Input: part model. Units: mm. Frame: model coordinates. Give positions to 0.01 mm unless a question says otherwise; leave off trailing zeros. Loops run counter-clockwise (first coordinate to the right, second up) from the corner with the lowest first, then second, coordinate; pieces in that order, holes last. Notation, with made-up numbers: (6, 66.25) - (35, 66.25) arc R20 ccw to (35, 75.25) - close; hole circle Ø5 at (50, 9). An arc over 180 degrees is marked (long way). Answer as a JSON object with one key per item and string values.
from build123d import *

# Parameters (mm, degrees)
BOSS_EXTRUDE2_DEPTH                          = 2
F_3_2_3_2_DIAMETER_HOLE1_D                   = 3.2
F_3_2_3_2_DIAMETER_HOLE2_D                   = 3.2
F_3_2_3_2_DIAMETER_HOLE3_D                   = 3.2
F_3_2_3_2_DIAMETER_HOLE5_D                   = 3.2
F_3_2_3_2_DIAMETER_HOLE5_DEPTH               = 10
F_3_2_3_2_DIAMETER_HOLE5_TIP                 = 0.96137699
CSK_FOR_M3_FLAT_COUNTERSUNK_HEAD_SCR_2_COUNT = 2
CSK_FOR_M3_FLAT_COUNTERSUNK_HEAD_SCR_2_PITCH = 78
CSK_FOR_M3_FLAT_COUNTERSUNK_HEAD_SCR_3_COUNT = 2
CSK_FOR_M3_FLAT_COUNTERSUNK_HEAD_SCR_3_PITCH = 110.308657865
FILLET1_R                                    = 3
M2_5X0_45_TAPPED_HOLE1_D                     = 2.05


with BuildPart() as part:
    # Sketch2 → Boss-Extrude2 (new body)
    with BuildSketch(Plane.ZY.offset(51.493641502)):
        Polygon((0.93465612, 3.45185693), (7.43465612, 3.45185693), (7.43465612, 86.45185693), (0.93465612, 86.45185693), (0.93465612, 92.95185693), (-82.06534388, 92.95185693), (-82.06534388, 86.45185693), (-88.56534388, 86.45185693), (-88.56534388, 3.45185693), (-82.06534388, 3.45185693), (-82.06534388, -3.04814307), (0.93465612, -3.04814307), align=None)
        Polygon((-71.56534388, 86.45185693), (-82.06534388, 75.95185693), (-82.06534388, 13.95185693), (-71.56534388, 3.45185693), (-9.56534388, 3.45185693), (0.93465612, 13.95185693), (0.93465612, 75.95185693), (-9.56534388, 86.45185693), align=None, mode=Mode.SUBTRACT)
    extrude(amount=BOSS_EXTRUDE2_DEPTH)

    # Sketch10 → CSK for M3 Flat Countersunk Head Screw3 (revolve, cut)
    with BuildSketch(Plane(origin=(-53.493641502, 5.95185693, -1.56534388), x_dir=(0, 0, 1), z_dir=(0, 1, 0))):
        Polygon((0, 0), (0, 2), (1.6, 2), (1.6, 1.65), (3.25, 0), align=None)
    revolve(axis=Axis((-59.843641502, 5.95185693, -1.56534388), (1, 0, 0)), mode=Mode.SUBTRACT)

    # Ø3.2 (3.2) Diameter Hole1 (through all)
    with Locations(Plane.ZY.offset(53.493641502)):
        with Locations((4.43465612, 6.95185693)):
            Hole(F_3_2_3_2_DIAMETER_HOLE1_D / 2)

    # Ø3.2 (3.2) Diameter Hole2 (through all)
    with Locations(Plane.ZY.offset(53.493641502)):
        with Locations((-2.56534388, -0.04814307)):
            Hole(F_3_2_3_2_DIAMETER_HOLE2_D / 2)

    # Ø3.2 (3.2) Diameter Hole3 (through all)
    with Locations(Plane.ZY.offset(53.493641502)):
        with Locations((-78.56534388, -0.04814307)):
            Hole(F_3_2_3_2_DIAMETER_HOLE3_D / 2)

    # Ø3.2 (3.2) Diameter Hole5
    with Locations(Plane(origin=(-53.493641502, 6.95185693, -85.56534388), x_dir=(0, 0, -1), z_dir=(-1, 0, 0))):
        with Locations((0, 0), (0, -76), (-7, -83), (-83, -83), (-90, -76)):
            Hole(F_3_2_3_2_DIAMETER_HOLE5_D / 2, depth=F_3_2_3_2_DIAMETER_HOLE5_DEPTH)
            with Locations((0, 0, -(F_3_2_3_2_DIAMETER_HOLE5_DEPTH + F_3_2_3_2_DIAMETER_HOLE5_TIP / 2))):  # 118° drill point
                Cone(0, F_3_2_3_2_DIAMETER_HOLE5_D / 2, F_3_2_3_2_DIAMETER_HOLE5_TIP, mode=Mode.SUBTRACT)

    # Sketch24 → CSK for M3 Flat Countersunk Head Screw5 (revolve, cut)
    with BuildSketch(Plane(origin=(-53.493641502, 5.95185693, -79.56534388), x_dir=(0, 0, 1), z_dir=(0, 1, 0))):
        Polygon((0, 0), (0, 2), (1.6, 2), (1.6, 1.65), (3.25, 0), align=None)
    csk_for_m3_flat_countersunk_head_screw5 = revolve(axis=Axis((-59.843641502, 5.95185693, -79.56534388), (1, 0, 0)), mode=Mode.SUBTRACT)

    # CSK for M3 Flat Countersunk Head Scr 2: CSK for M3 Flat Countersunk Head Screw5 ×2
    with Locations(*[(0, i * CSK_FOR_M3_FLAT_COUNTERSUNK_HEAD_SCR_2_PITCH, 0) for i in range(1, CSK_FOR_M3_FLAT_COUNTERSUNK_HEAD_SCR_2_COUNT)]):
        add(csk_for_m3_flat_countersunk_head_screw5, mode=Mode.SUBTRACT)

    # CSK for M3 Flat Countersunk Head Scr 3: CSK for M3 Flat Countersunk Head Screw5 ×2
    with Locations(*[Vector(0, 0.7071067811865477, 0.7071067811865474) * (i * CSK_FOR_M3_FLAT_COUNTERSUNK_HEAD_SCR_3_PITCH) for i in range(1, CSK_FOR_M3_FLAT_COUNTERSUNK_HEAD_SCR_3_COUNT)]):
        add(csk_for_m3_flat_countersunk_head_screw5, mode=Mode.SUBTRACT)

    # Fillet1
    fillet1_edges = [part.edges().sort_by_distance(p)[0] for p in [
        (-52.493641502, 86.45185693, -9.56534388),
        (-52.493641502, 86.45185693, -71.56534388),
        (-52.493641502, 75.95185693, -82.06534388),
        (-52.493641502, 13.95185693, -82.06534388),
        (-52.493641502, 3.45185693, -71.56534388),
        (-52.493641502, 3.45185693, -9.56534388),
        (-52.493641502, 13.95185693, 0.93465612),
        (-52.493641502, 75.95185693, 0.93465612),
    ]]
    fillet(fillet1_edges, radius=FILLET1_R)

    # M2.5x0.45 Tapped Hole1 (through all)
    with Locations(Plane(origin=(-53.493641502, 89.45185693, -40.56534388), x_dir=(0, 0, -1), z_dir=(-1, 0, 0))):
        with Locations((0, 0), (44.5, 44.5), (0, 89), (-44.5, 44.5)):
            Hole(M2_5X0_45_TAPPED_HOLE1_D / 2)


solid = part.part
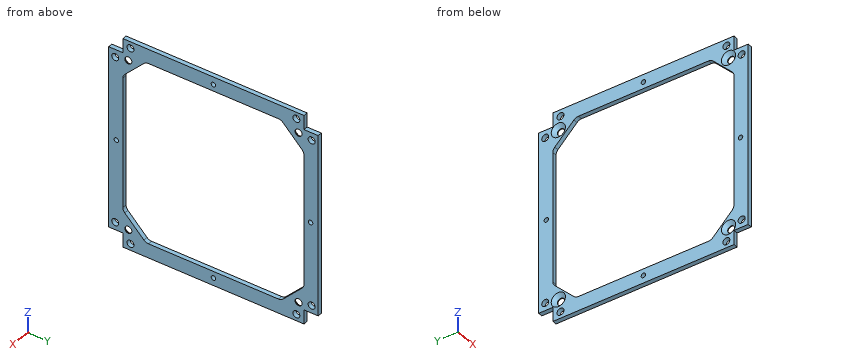
Item 1: Cut plane A-A (z = -12). Return loops of the section in (x, y).
Geometry check:
{"outline": "(-53.49, -3.05) - (-51.49, -3.05) - (-51.49, 3.45) - (-53.49, 3.45) - close; (-53.49, 86.45) - (-51.49, 86.45) - (-51.49, 92.95) - (-53.49, 92.95) - close"}
Item 2: Material intervals for line 1 (Y direction, x = -52.9, z = -31.5); line 2 (Z direction, x = -51.7, y = 28); line 3 (Y direction, x = -52.75, z = -78), sorted ascending. Write a range as [from, to].
Geometry check:
{"line 1": "y = [-3.05, 3.45], [86.45, 92.95]", "line 2": "z = [-88.57, -82.07], [0.93, 7.43]", "line 3": "y = [-3.05, -1.54], [1.45, 3.99], [7.91, 9.89], [80.02, 81.99], [85.91, 88.46], [91.45, 92.95]"}
Item 3: Cut plane C-C (x = -52.85). Give the number of separate pieces and of enclosed holes in the cut face, then the cut area to 3 significant figures.
Geometry check:
{"separate pieces": "1", "enclosed holes": "17", "area": "2,220 mm2"}
Item 4: Cut plane B-B (y = 25). Return loops of the section in (x, z).
Geometry check:
{"outline": "(-53.49, -88.57) - (-51.49, -88.57) - (-51.49, -82.07) - (-53.49, -82.07) - close; (-53.49, 0.93) - (-51.49, 0.93) - (-51.49, 7.43) - (-53.49, 7.43) - close"}
Item 5: Contact query for flat-ended pins moving along their axis: P1, Ø1, axis at x = -53, y = 89.5, coming from the +Z side; P2, Ø3.5, axis at y = -0.05, z = -2.57, coming from the +X side. Output: stop coordinate, or through.
Geometry check:
{"P1": "stops at z = 0.93", "P2": "stops at x = -51.49"}
